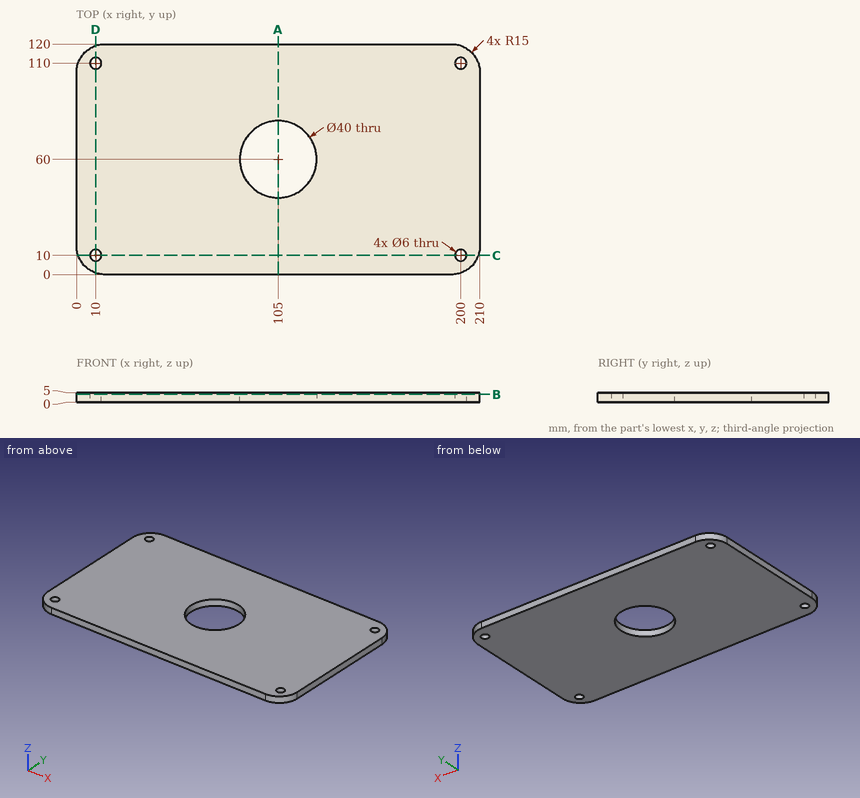
Input: dimensioned drawing with shaded views. Units: mm. Origin: part minimum x, y, z. Coordinates: 2 decimals unless noted, no trailing zeros. Order: outer loops, then holes, each group sorted by start corner. A loop starts at its lowest first (then second) coordinate and runs counter-clockwise, first axis right, second up.
(1) Section query B-B (z = 4.05). Return the cut outline in (x, y).
(2) Section query D-D (x = 10). Return the cut outline in (y, z).
(3) First-contact query: pin 1 (5 mm diameter, centred on x = 10, y = 110, fed in from -Z); pin 2 (8 mm diameter, centred on x = 200, y = 10, fed in from -Z). Flat tips, straight axial feed; report the tip coordinate or a pass-through.
(4) Section query C-C (y = 10). Return the cut outline in (x, z), plus the area to 3 significant figures.
(5) Material intervals for probe 1 along X at (y, z) = (112, 4.7); probe 2 along Y at (x, z) = (10, 1.65); probe 3 along X at (y, z) = (70, 1.2), sorted ascending.
(6) Section query A-A (x = 105). Return the cut outline in (y, z), plus the area to 3 significant figures.
Solution:
1. outline: (0, 15) arc R15 ccw to (15, 0) - (195, 0) arc R15 ccw to (210, 15) - (210, 105) arc R15 ccw to (195, 120) - (15, 120) arc R15 ccw to (0, 105) - close; hole circle Ø6 at (10, 10); hole circle Ø6 at (10, 110); hole circle Ø40 at (105, 60); hole circle Ø6 at (200, 10); hole circle Ø6 at (200, 110)
2. outline: (0.86, 0) - (7, 0) - (7, 5) - (0.86, 5) - close; (13, 0) - (107, 0) - (107, 5) - (13, 5) - close; (113, 0) - (119.14, 0) - (119.14, 5) - (113, 5) - close
3. pin 1: passes through
3. pin 2: stops at z = 0
4. outline: (0.86, 0) - (7, 0) - (7, 5) - (0.86, 5) - close; (13, 0) - (197, 0) - (197, 5) - (13, 5) - close; (203, 0) - (209.14, 0) - (209.14, 5) - (203, 5) - close
4. area: 981 mm2
5. probe 1: x = 1.73 to 7.76, 12.24 to 197.76, 202.24 to 208.27
5. probe 2: y = 0.86 to 7, 13 to 107, 113 to 119.14
5. probe 3: x = 0 to 87.68, 122.32 to 210
6. outline: (0, 0) - (40, 0) - (40, 5) - (0, 5) - close; (80, 0) - (120, 0) - (120, 5) - (80, 5) - close
6. area: 400 mm2
